Read the model definition and answer for the solid it produces. Units are mm, in the model's axes. Face numbers are marked on the shaded views. A direction names the side the tool comes from. Coordinates: 2 decimals unless noted, no trailing zeros. Order: outer loops, then holes, each group sorted by start corner. A loop starts at its lowest first (then second) coordinate and runs counter-clockwise, first axis right, second up.
Autodesk Inventor part; units mm, degrees
ref_plane "РабПлоскость1" through (22.5, 0, 0) normal (1, 0, 0) x (0, 1, 0)
ref_plane "YZ Plane" through (0, 0, 0) normal (1, 0, 0) x (0, 1, 0)
ref_plane "XZ Plane" through (0, 0, 0) normal (0, 1, 0) x (-1, 0, 0)
sketch "Эскиз1" plane through (0, 0, 0) normal (0, 1, 0) x (-1, 0, 0)
  circle A0 centre (0, 0) radius 22.5
  dimension "d0" = 45
extrude "Выдавливание1" add sketch "Эскиз1" along normal blind 55
sketch "Эскиз2" plane through (0, 0, 0) normal (0, -1, 0) x (1, 0, 0)
  circle A0 centre (0, 0) radius 22.5
  point P0 (22.5, 0)
ref_plane "РабПлоскость1" through (22.5, 0, 0) normal (1, 0, 0) x (0, 1, 0)
sketch "Эскиз3" plane through (22.5, 0, 0) normal (1, 0, 0) x (0, 1, 0)
  line L0 (0, 0) -> (12.5, 0)
  line L1 (12.5, 0) -> (17.5, 0)
  circle A0 centre (15, 0) radius 2.5
  dimension "d3" = 12.5
  dimension "d4" = 5
hole "Отверстие1" at (22.5, 15, 0) direction (-1, 0, 0) diameter 4.134 depth 10 tip angle 118
sketch "Эскиз4" plane through (0, 55, 0) normal (0, 1, 0) x (1, 0, 0)
  point P0 (0, 0)
  point P1 (0, 0)
hole "Отверстие2" at (0, 55, 0) direction (0, -1, 0) diameter 13.3762 depth 20
sketch "Эскиз5" plane through (0, 0, 0) normal (0, -1, 0) x (1, 0, 0)
  circle A0 centre (0, 0) radius 8
  dimension "d27" = 16
extrude "Выдавливание2" cut sketch "Эскиз5" against normal blind 4
properties part number "17701729.304517.015"
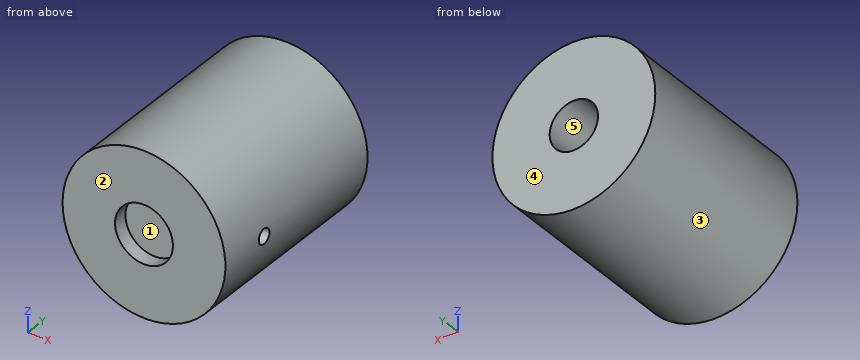
1) Straight lines are drawn through the part: line 1 (Z direction, x = 0, y = 1.85); line 2 (X direction, y = 39, z = 0); line 3 (Z direction, x = 15, y = 15). For each, find the intervals that lie inside material, in ascending order.
A:
line 1: z = -22.5 to -8, 8 to 22.5
line 2: x = -22.5 to -6.69, 6.69 to 22.5
line 3: z = -16.77 to -2.07, 2.07 to 16.77
2) A cutting plane is placed at C-C, the plane x = 17. Determine the outline of the cut face in (y, z).
A:
outline: (0, -14.74) - (55, -14.74) - (55, 14.74) - (0, 14.74) - close; hole circle Ø4.13 at (15, 0)
3) Flat-ended cylindrical pins translate along their axes: pin 1 Ø5 at (y, z) = (12, -5.5) entering from +X; pin 2 Ø1.5 at (x, y) = (1, 30.5) entering from -Z; pin 3 Ø1 at (x, y) = (2, 16) entering from +Z. Find the tip coordinate at first contact, or state that the pin passes through.
A:
pin 1: stops at x = 22.3
pin 2: stops at z = -22.5
pin 3: stops at z = 22.45
4) Determine the mould class of the marked faces 1, 2 and 3 for opening direction X: pulls with the +X half, pulls with the -X half, needs draft (parallel to the pull), parting line crosses it, or undercut.
A:
face 1: undercut
face 2: needs draft
face 3: parting line crosses it
5) A cutting plane is placed at B-B, the plane y = 47.5. Determine the outline of the cut face in (x, z), and give its area (3 significant figures).
A:
outline: circle Ø45 at (0, 0); hole circle Ø13.38 at (0, 0)
area: 1,450 mm2
6) A cutting plane is placed at D-D, the plane z = -4. Determine the outline of the cut face in (x, y).
A:
outline: (-22.14, 0) - (-6.93, 0) - (-6.93, 4) - (6.93, 4) - (6.93, 0) - (22.14, 0) - (22.14, 55) - (5.36, 55) - (5.36, 35) - (-5.36, 35) - (-5.36, 55) - (-22.14, 55) - close
7) Which of the six approach directions +Z, -Z, +X, -X, +Y, -Y give full straight-line access (tool end or side, diameter ignored) to the marked faces 4 and 5?
A:
face 4: +Z, -Z, +X, -X, +Y
face 5: +Y
8) A cutting plane is placed at A-A, the plane x = 0. Determine the outline of the cut face in (y, z).
A:
outline: (0, -22.5) - (55, -22.5) - (55, -6.69) - (35, -6.69) - (35, 6.69) - (55, 6.69) - (55, 22.5) - (0, 22.5) - (0, 8) - (4, 8) - (4, -8) - (0, -8) - close
